```python
from build123d import *

# Parameters (mm, degrees)
SKETCH2_R           = 2.25
BOSS_EXTRUDE1_DEPTH = 3


with BuildPart() as part:
    # Sketch2 → Boss-Extrude1 (new body)
    with BuildSketch(Plane(origin=(54.951104055, -12.928200351, 0), x_dir=(1, 0, 0), z_dir=(0, 0, 1))):
        Polygon((150.346314429, -129.315759544), (150.346314429, -171.376869313), (85.688434657, -236.034749085), (-85.688434657, -64.657879772), (-21.030554884, 0), (21.030554884, 0), align=None)
        with Locations((-3.979949748, -14.5)):
            Circle(SKETCH2_R, mode=Mode.SUBTRACT)
        with Locations((3.979949748, -14.5)):
            Circle(SKETCH2_R, mode=Mode.SUBTRACT)
        with Locations((135.846314429, -154.326264177)):
            Circle(SKETCH2_R, mode=Mode.SUBTRACT)
        with Locations((135.846314429, -146.36636468)):
            Circle(SKETCH2_R, mode=Mode.SUBTRACT)
    extrude(amount=BOSS_EXTRUDE1_DEPTH)

    # Mirror1: part across plane


with BuildPart() as part_1:
    add(part.part)
    add(part.part.mirror(Plane(origin=(140.639538712, -248.962949436, 3), x_dir=(0, 0, 1), z_dir=(0.707106781186551, 0.7071067811865441, 0))))


solid = part_1.part
```
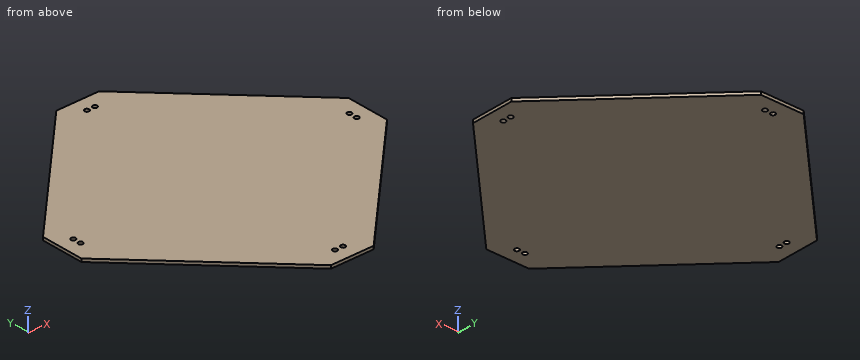
Input: part model. Units: mm. Frame: model coordinates. Round coordinates to 2 decimals unless told otherwise and drop trailing zeros. Order: outer loops, then holes, each group sorted by start corner. A loop starts at its lowest first (then second) coordinate and runs counter-clockwise, first axis right, second up. Notation, with made-up numbers: (71.25, 89.25) - (126.25, 89.25) arc R26 ccw to (126.25, 114.25) - close; hole circle Ø1 at (46.5, -32.75). An arc over 180 degrees is marked (long way). One line per question, with ' | ' between items. Start each with the question number.
1) Ray query, probe 1 along Y at (x, z) = (16, 2.1); probe 2 along Y at (x, z) = (130.5, 1.25); probe 3 along X at (y, z) = (-100, 1.3). Return the intervals inside material, ascending.
2) Cut plane C-C, the plane x = -15. Return the cut outline in (y, z), then the cut area to 3 significant figures.
3) Cut plane A-A, the plane z = 0.45. Give the number of separate pieces and of enclosed holes in the cut face, then the cut area to 3 significant figures.
4) Cut plane B-B, the plane y = -286.5. Return the cut outline in (x, z), then the cut area to 3 significant figures.
Worked out:
1) probe 1: y = -295.7 to -30.85 | probe 2: y = -259.1 to -67.45 | probe 3: x = -53.15 to 163.05
2) outline: (-264.7, 0) - (-61.85, 0) - (-61.85, 3) - (-264.7, 3) - close | area: 609 mm^2
3) separate pieces: 1 | enclosed holes: 8 | area: 56,800 mm^2
4) outline: (6.8, 0) - (103.1, 0) - (103.1, 3) - (6.8, 3) - close | area: 289 mm^2
